Geometry check sheet. Reference: drawing and pictorial views, mm from the part's lowest x, y, z. A direction names the side the tool comes from. Give positions to 0.01 mm unless a question says otherwise; leave off trailing zeros. Order: outer loops, then holes, each group sorted by start corner. A loop starts at its lowest first (then second) coordinate and runs counter-clockwise, first axis right, second up. Notation, with made-up numbers: M -2.5,30.5 L 45.5,30.5 A7 ccw 45.5,39.5 Z; hole C 18.5,-34.75 d11. An arc over 180 degrees is marked long. Answer as CSV lines item,"result".
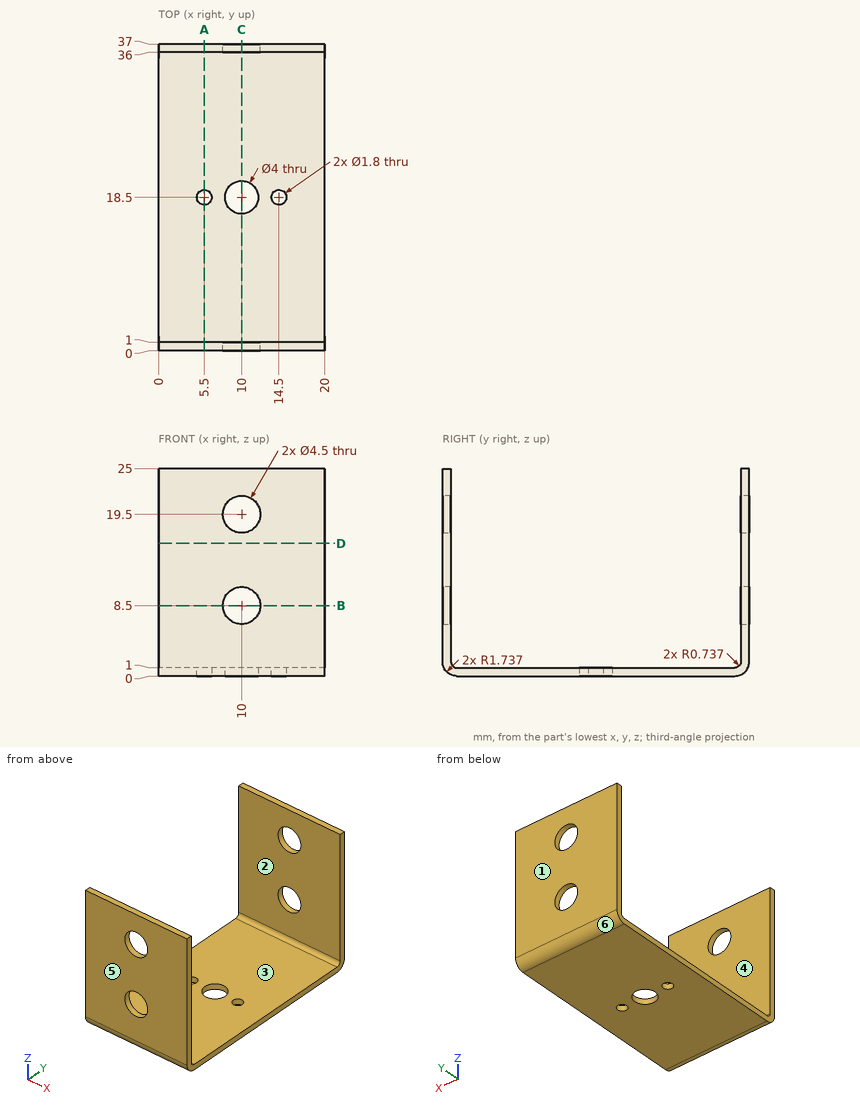
(1) Gauge pin test, flat ends, axial feed: P1, Ø4, axis at x = 7.5, y = 23.5, coming from the -Z side; P2, Ø1.1, axis at x = 5.5, y = 18.5, coming from the +Z side; P3, Ø2, axis at x = 9, y = 13, coming from the +Z side. Record the tip position at first contact, or that the pin passes through.
The answers:
P1,"stops at z = 0"
P2,"passes through"
P3,"stops at z = 1"
(2) Section check A-A on x = 5.5. Enter the section's corners in (y, z).
The answers:
outline,"M 0,1.74 A1.74 ccw 1.74,0 L 17.6,0 L 17.6,1 L 1.74,1 A0.74 cw 1,1.74 L 1,25 L 0,25 Z; M 19.4,0 L 35.26,0 A1.74 ccw 37,1.74 L 37,25 L 36,25 L 36,1.74 A0.74 cw 35.26,1 L 19.4,1 Z"
(3) Material ranges on line 1 (X direction, y = 0.35, z = 8.5); line 2 (Y direction, x = 9.75, z = 2); line 3 (Z direction, x = 9, y = 6), recorded low to high.
The answers:
line 1,"x = 0 to 7.75, 12.25 to 20"
line 2,"y = 0 to 1, 36 to 37"
line 3,"z = 0 to 1"
(4) Section check B-B on z = 8.5. Enter the section's corners in (x, y).
The answers:
outline,"M 0,0 L 7.75,0 L 7.75,1 L 0,1 Z; M 0,36 L 7.75,36 L 7.75,37 L 0,37 Z; M 12.25,0 L 20,0 L 20,1 L 12.25,1 Z; M 12.25,36 L 20,36 L 20,37 L 12.25,37 Z"
(5) Tool access check on the marked faces 1 and 2. Record the directions out of +Z, -Z, +X, -X, +Y, -Y that give a thin tool (end or side, any length) a straight path to the whole face; none if there is none.
The answers:
face 1,"+Z, -Z, +X, -X, +Y"
face 2,"+Z, +X, -X"
(6) Draft check along Y on the marked faces 3, 4, 5 and 6. Enter one of: +Y half, -Y half, draft (parallel to the pull), parting line (faces both ways), or undercut.
The answers:
face 3,"undercut"
face 4,"undercut"
face 5,"-Y half"
face 6,"+Y half"
(7) Section check C-C on x = 10. State how many separate pieces and enclosed holes the cut face has.
The answers:
separate pieces,"6"
enclosed holes,"0"
(8) Section check D-D on z = 16. Enter the section's corners in (x, y).
The answers:
outline,"M 0,0 L 20,0 L 20,1 L 0,1 Z; M 0,36 L 20,36 L 20,37 L 0,37 Z"
